Solid Edge part; units mm, degrees
sketch "Sketch1" plane through (0, 0, 0) normal (0, 0, 1) x (1, 0, 0)
  line L0 (-118.5746, 131.2039) -> (-118.5746, -68.7961)
  line L1 (-118.5746, -68.7961) -> (6.8792, -68.7961)
  line L2 (6.8792, -68.7961) -> (6.8792, 131.2039)
  line L3 (6.8792, 131.2039) -> (-118.5746, 131.2039)
  line L4 (-118.5746, 131.2039) -> (81.4254, 131.2039)
  line L5 (81.4254, 131.2039) -> (81.4254, 231.2039)
  line L6 (81.4254, 231.2039) -> (-118.5746, 231.2039)
  line L7 (-118.5746, 231.2039) -> (-118.5746, 131.2039)
  dimension "D1" = 81.4254
  dimension "D2" = 118.5746
  dimension "D3" = 118.5746
extrude "Protrusion1" add sketch "Sketch1" along normal blind 20
sketch "Sketch2" plane through (-18.5746, 131.2039, 20) normal (0, 0, 1) x (1, 0, 0)
  circle A0 centre (0, 55) radius 20
extrude "Cutout1" cut sketch "Sketch2" against normal through all
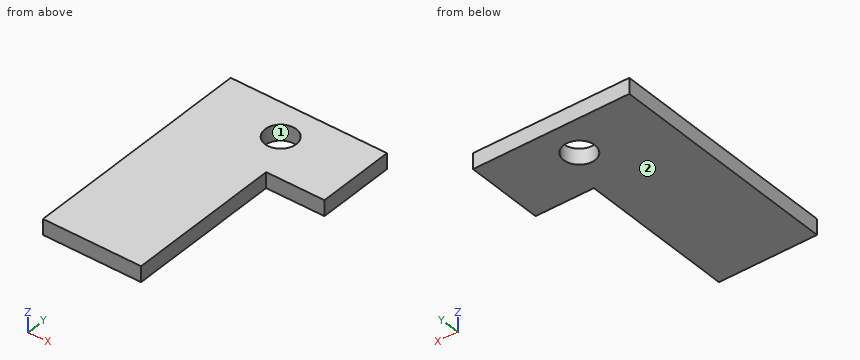
Geometry: final body of the model. Coordinates: model frame, mm. Face numbers are marked on the shaded views. Coordinates: 2 decimals unless noted, no trailing zeros. Order: outer loops, then holes, each group sorted by start corner. A loop starts at its lowest first (then second) coordinate and runs counter-clockwise, first axis right, second up. Notation, with made-up numbers: M -5,22 L 1,22 A17 cw 1,41 Z; hole C 21.25,-9 d6. An arc over 180 degrees is marked long. Answer as CSV lines item,"result".
Q1. Draft query along X for the marked faces 1 and 2. Return one class per face: pulls with the +X half, pulls with the -X half, needs draft (parallel to the pull), parting line crosses it, or undercut.
Answers:
face 1,"undercut"
face 2,"needs draft"
Q2. Section A-A on x = -16.5. Return the cut outline in (y, z).
Answers:
outline,"M -68.8,0 L 166.31,0 L 166.31,20 L -68.8,20 Z; M 206.1,0 L 231.2,0 L 231.2,20 L 206.1,20 Z"
Q3. Section B-B on y = 200. Return the cut outline in (x, z).
Answers:
outline,"M -118.57,0 L -33.05,0 L -33.05,20 L -118.57,20 Z; M -4.09,0 L 81.43,0 L 81.43,20 L -4.09,20 Z"
Q4. Line query: probe 1 along Y at (x, z) = (7, 5); probe 2 along X at (y, z) = (19, 2.5); probe 3 along X at (y, z) = (182.5, 13.5). Output: solid intervals per line, ascending. Write a range as [from, to].
Answers:
probe 1,"y = [131.2, 231.2]"
probe 2,"x = [-118.57, 6.88]"
probe 3,"x = [-118.57, -38.23], [1.08, 81.43]"
Q5. Section D-D on x = 60. Return the cut outline in (y, z).
Answers:
outline,"M 131.2,0 L 231.2,0 L 231.2,20 L 131.2,20 Z"
Q6. First-contact query: P1, Ø10, axis at y = 73.5, z = 5, coming from the +X side; P2, Ø6, axis at x = 32, z = 5, coming from the -Y side. Flat tips, straight axial feed; report the tip coordinate or a pass-through.
Answers:
P1,"stops at x = 6.88"
P2,"stops at y = 131.2"
Q7. Section C-C on z = 7. Return the cut outline in (x, y).
Answers:
outline,"M -118.57,-68.8 L 6.88,-68.8 L 6.88,131.2 L 81.43,131.2 L 81.43,231.2 L -118.57,231.2 Z; hole C -18.57,186.2 d40"
